CAD build for the part. Positions are in the model's coordinates, mm. Face numbers are marked on the shaded views. A direction names the side the tool comes from. Round coordinates to 2 decimals unless told otherwise and drop trailing zeros. Order: outer loops, then holes, each group sorted by start corner. A loop starts at its lowest first (then second) coordinate and runs counter-clockwise, first axis right, second up. Notation, with made-up numbers: M 47.25,-11 L 104.25,-11 A14 ccw 104.25,4 Z; hole C 79,29.25 d2. An arc over 180 degrees is marked long. Put each result on its own line as item: value.
```python
from build123d import *

# Parameters (mm, degrees)
F0_W     = 101.6
F0_H     = 50.8
F1_DEPTH = 406.4
F2_W     = 101.6
F2_H     = 25.4
F3_DEPTH = 50.8
F4_W     = 101.6
F4_H     = 25.4
F5_DEPTH = 50.8
F6_R     = 3.175
F7_DEPTH = 50.801
F8_R     = 6.35
F9_DEPTH = 6.35
F9_TAPER = 30


with BuildPart() as f1:
    # F0 (on Top) → F1 (new body)
    with BuildSketch(Plane.XY):
        Rectangle(F0_W, F0_H)
    extrude(amount=F1_DEPTH)

    # F2 (on face) → F3 (cut)
    with BuildSketch(Plane.XY.offset(406.4)):
        with Locations((0, -12.7)):
            Rectangle(F2_W, F2_H)
    extrude(amount=-F3_DEPTH, mode=Mode.SUBTRACT)

    # F4 (on face) → F5 (cut)
    with BuildSketch(Plane(origin=(0, 0, 0), x_dir=(1, 0, 0), z_dir=(0, 0, -1))):
        with Locations((0, 12.7)):
            Rectangle(F4_W, F4_H)
    extrude(amount=-F5_DEPTH, mode=Mode.SUBTRACT)

    # F6 (on face) → F7 (cut, through all)
    with BuildSketch(Plane(origin=(0, 25.4, 0), x_dir=(-1, 0, 0), z_dir=(0, 1, 0))):
        with Locations((0, 381)):
            Circle(F6_R)
        with Locations((0, 25.4)):
            Circle(F6_R)
    extrude(amount=-F7_DEPTH, mode=Mode.SUBTRACT)

    # F8 (on face) → F9 (cut)
    with BuildSketch(Plane(origin=(0, 25.4, 0), x_dir=(-1, 0, 0), z_dir=(0, 1, 0))):
        with Locations((0, 381)):
            Circle(F8_R)
        with Locations((0, 25.4)):
            Circle(F8_R)
    extrude(amount=-F9_DEPTH, taper=F9_TAPER, mode=Mode.SUBTRACT)


solid = f1.part
```
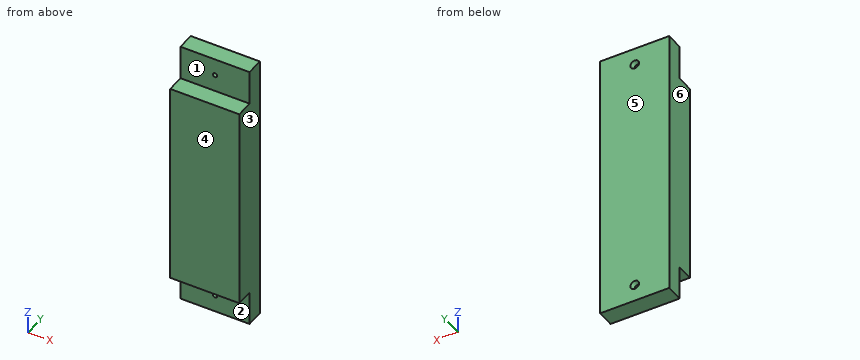
Item 1: Pin check, flat tips, straight feed: P1, Ø15, axis at x = -9.5, z = 377.5, coming from the -Y side; P2, Ø12.5, axis at x = 11.5, y = -9.5, coming from the -Z side; P3, Ø3, axis at x = 20, y = -20, coming from the +Z side. Stop position of each tip, or through.
Answers below:
P1: y = 0
P2: z = 50.8
P3: z = 355.6
Item 2: Probe line 1 along Z through (x, y) = (0, 5) (3 decimals); line 2 along X through (y, z) = (15, 25.4) (3 decimals); line 3 along X through (y, z) = (15, 25). List the from-to ranges inside material, lowest first. Write a range as [from, to].
Answers below:
line 1: [0, 22.225], [28.575, 377.825], [384.175, 406.4]
line 2: [-50.8, -3.175], [3.175, 50.8]
line 3: [-50.8, -3.15], [3.15, 50.8]
Item 3: Mould opens along Y. For the marked faces 4, 5 and 6 say: pulls with the +Y half, pulls with the -Y half, needs draft (parallel to the pull), parting line crosses it, or undercut.
Answers below:
face 4: pulls with the -Y half
face 5: pulls with the +Y half
face 6: needs draft
Item 4: Band-saw the part on A-A on x = 25.5. Give the cut face in (y, z), and give its area (3 significant figures).
Answers below:
outline: M -25.4,50.8 L 0,50.8 L 0,0 L 25.4,0 L 25.4,406.4 L 0,406.4 L 0,355.6 L -25.4,355.6 Z
area: 18,100 mm²
Item 5: Tool access for the marked faces 1, 2 and 3: list every direction of +Z, -Z, +X, -X, +Y, -Y with a clear straight run to the whole face (end or side of a thin tool).
Answers below:
face 1: +Z, +X, -X, -Y
face 2: -Z, +X, -X, -Y
face 3: +Z, -Z, +X, +Y, -Y
Item 6: Band-saw the part on B-B on y = -11. Give the cut face in (x, z), and give its area (3 significant figures).
Answers below:
outline: M -50.8,50.8 L 50.8,50.8 L 50.8,355.6 L -50.8,355.6 Z
area: 31,000 mm²
